For this review, use the dimensioned drawing (mm, ordinates from the lowest corner) and the shaded views. A direction names the side the tool comes from. Round coordinates to 2 decimals unless told otherwise and drop trailing zeros. Loops run counter-clockwise (first coordinate to the right, second up) from the corner with the lowest first, then second, coordinate; pieces in that order, holes last. Notation, with made-up numbers: M -34,-8 L -22,-8 A36 cw -22,31 Z; hole C 42.25,60.25 d8. An arc over 180 degrees is marked long. Answer as a JSON object with one key per item and string values. Group by question number.
Item 1: Consider section D-D (z = 3.7). Give the boundary of the cut face in (x, y).
Item 2: To check wall thickness, follow line 1 (Y direction, x = 0.7, z = 1.85); line 2 (Z direction, x = 1.35, y = 4.5); line 3 (Z direction, x = 0.55, y = 4.5). State the ranges of each line that lie inside material, in increasing order.
Item 3: The part is to be moulded in two halves that separate along Z. For the marked faces 1, 2, 3 and 4, say which applies: +Z half, -Z half, draft (parallel to the pull), parting line (faces both ways), or undercut.
Item 4: Insertion check: P1, Ø1.6, axis at y = 13.5, z = 2, coming from the +X side; P2, Ø0.6, axis at x = 5.5, z = 2, coming from the -Y side; P3, Ø0.6, axis at x = 5.5, z = 4, coming from the +Y side. Each pin has a flat end and moves straight along its axis. Give the tip position at first contact, or say it passes through.
Item 5: Consider section B-B (z = 1.65). Give the boundary of the cut face in (x, y).
Item 6: Tool access review of the marked faces 5, 6, 7 and 8: name each direction out of +Z, -Z, +X, -X, +Y, -Y from which nothing blocks a thin tool from reaching the whole face with its end or side.
Item 7: Consider section A-A (y = 2.75). Give the boundary of the cut face in (x, z), and give its area (4 significant figures).
Item 8: Consider section C-C (x = 4.75). Give the boundary of the cut face in (y, z), and give its area (3 significant figures).
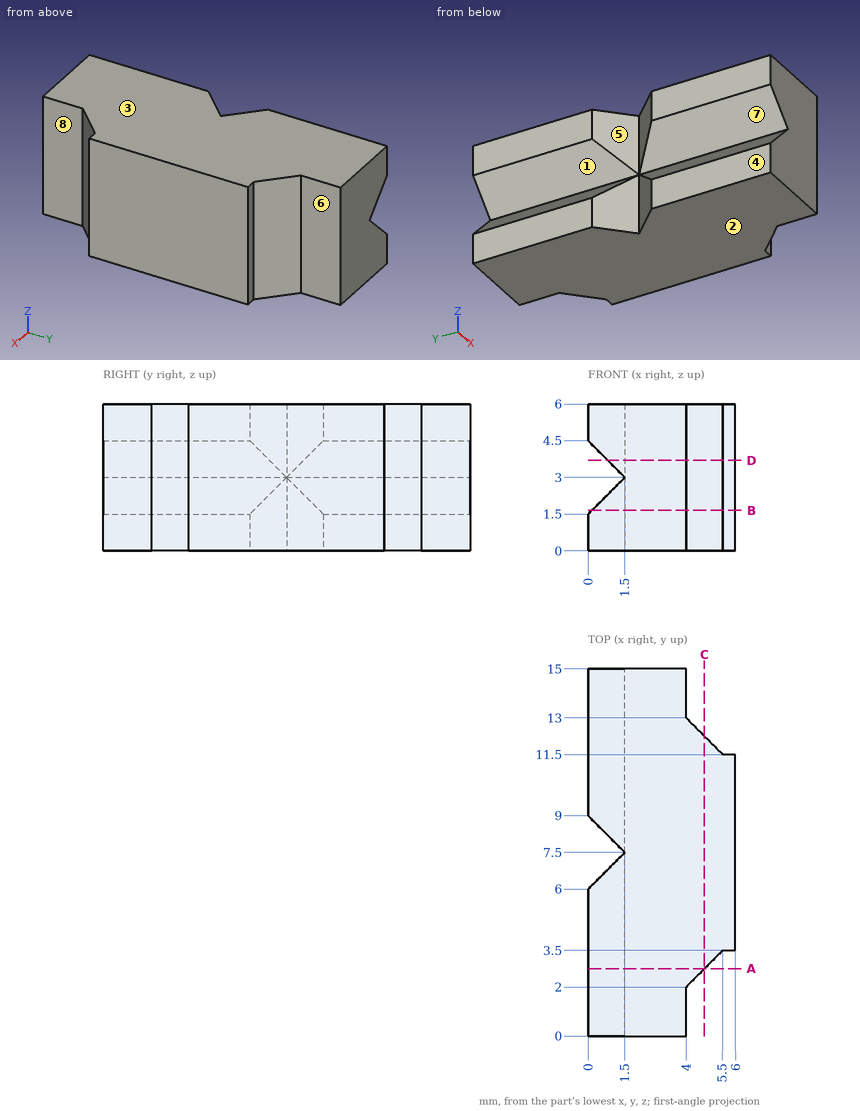
Geometry results:
{
 "1": {"outline": "M 0.8,0 L 4,0 L 4,2 L 5.5,3.5 L 6,3.5 L 6,11.5 L 5.5,11.5 L 4,13 L 4,15 L 0.8,15 L 0.8,8.2 L 1.5,7.5 L 0.8,6.8 Z"},
 "2": {"line 1": "y = 0 to 6.7, 8.3 to 15", "line 2": "z = 0 to 2.85, 3.15 to 6", "line 3": "z = 0 to 2.05, 3.95 to 6"},
 "3": {"face 1": "undercut", "face 2": "-Z half", "face 3": "+Z half", "face 4": "draft"},
 "4": {"P1": "stops at x = 4.3", "P2": "stops at y = 3.2", "P3": "stops at y = 11.8"},
 "5": {"outline": "M 0.15,0 L 4,0 L 4,2 L 5.5,3.5 L 6,3.5 L 6,11.5 L 5.5,11.5 L 4,13 L 4,15 L 0.15,15 L 0.15,8.85 L 1.5,7.5 L 0.15,6.15 Z"},
 "6": {"face 5": "+Z, -Z, -X", "face 6": "+Z, -Z, +X, +Y", "face 7": "-X, +Y, -Y", "face 8": "+Z, -Z, +X, -Y"},
 "7": {"outline": "M 0,0 L 4.75,0 L 4.75,6 L 0,6 L 0,4.5 L 1.5,3 L 0,1.5 Z", "area": "26.25 mm^2"},
 "8": {"outline": "M 2.75,0 L 12.25,0 L 12.25,6 L 2.75,6 Z", "area": "57.0 mm^2"}
}
